Autodesk Inventor part; units mm, degrees
ref_plane "YZ Plane" through (0, 0, 0) normal (1, 0, 0) x (0, 1, 0)
ref_plane "XZ Plane" through (0, 0, 0) normal (0, 1, 0) x (-1, 0, 0)
ref_plane "XY Plane" through (0, 0, 0) normal (0, 0, 1) x (1, 0, 0)
sketch "スケッチ1" plane through (0, 0, 0) normal (0, 0, 1) x (1, 0, 0)
  circle A0 centre (0, 0) radius 30
  circle A1 centre (0, 0) radius 28
  dimension "d0" = 60
  dimension "d21" = 2
extrude "押し出し1" add sketch "スケッチ1" along normal blind 60
sketch "スケッチ6" plane through (0, 0, 0) normal (0, 0, -1) x (-1, 0, 0)
  circle A0 centre (0, 0) radius 28
extrude "押し出し5" add sketch "スケッチ6" against normal blind 2
sketch "スケッチ7" plane through (0, 0, 0) normal (0, 0, -1) x (-1, 0, 0)
  line L0 (0, 0) -> (-30, 0)
  circle A0 centre (0, 0) radius 30
  line L1 (0, 0) -> (0, 30)
  point P0 (-10, -15)
  point P1 (-10, 15)
  point P2 (10, -15)
  point P3 (10, 15)
  dimension "d24" = 20
  dimension "d25" = 30
hole "穴2" at (10, -15, 0) at (10, 15, 0) at (-10, -15, 0) at (-10, 15, 0) direction (0, 0, 1) diameter 3.5 end through all
properties part number "筒"
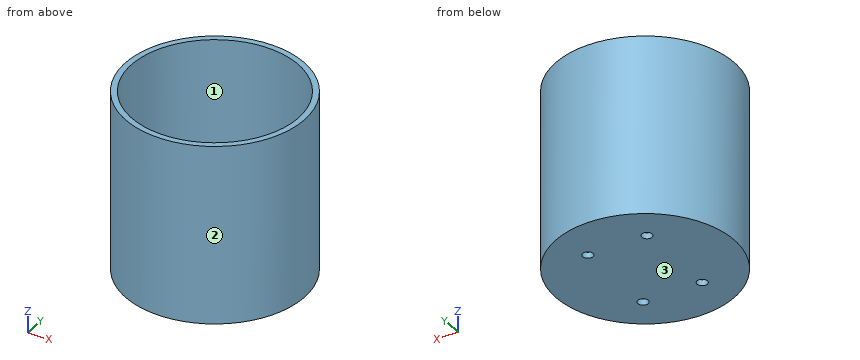
Can you work these out from the model? Positions are in its coordinate system, mm. Face numbers are marked on the shaded views. Coordinates: 2 decimals unless noted, no trailing zeros. Order: outer loops, then holes, each group sorted by start corner. A loop starts at its lowest first (then second) coordinate and runs counter-clockwise, first axis right, second up. Notation, with made-up numbers: (34, -10) - (68, -10) arc R13 ccw to (68, -3) - close; hole circle Ø7 at (15.5, 11.25). An arc over 180 degrees is marked (long way). Answer in a Markdown table with one row per item.
1. If I drill on line 1 along Y through (x, z) = (-10, 1.35); line 2 along X through (y, z) = (15, 0.7); line 3 along Z through (x, y) = (13.5, -17), over which ranges is the centre line in solid material (lowest first)?
Reply:
| item | result |
|---|---|
| line 1 | y = -28.28 to -16.75, -13.25 to 13.25, 16.75 to 28.28 |
| line 2 | x = -25.98 to -11.75, -8.25 to 8.25, 11.75 to 25.98 |
| line 3 | z = 0 to 2 |
2. Suppose I cut it at D-D (z = 53.5). Please give me the cut outline in (x, y), and give its area (3 significant figures).
Reply:
| item | result |
|---|---|
| outline | circle Ø60 at (0, 0); hole circle Ø56 at (0, 0) |
| area | 364 mm^2 |
3. Suppose I cut it at A-A (x = 0). Please give me the cut outline in (y, z), and give its area (3 significant figures).
Reply:
| item | result |
|---|---|
| outline | (-30, 0) - (30, 0) - (30, 60) - (28, 60) - (28, 2) - (-28, 2) - (-28, 60) - (-30, 60) - close |
| area | 352 mm^2 |
4. Suppose I cut it at B-B (x = 10). Please give me the cut outline in (y, z).
Reply:
| item | result |
|---|---|
| outline | (-28.28, 0) - (-16.75, 0) - (-16.75, 2) - (-26.15, 2) - (-26.15, 60) - (-28.28, 60) - close; (-13.25, 0) - (13.25, 0) - (13.25, 2) - (-13.25, 2) - close; (16.75, 0) - (28.28, 0) - (28.28, 60) - (26.15, 60) - (26.15, 2) - (16.75, 2) - close |
5. If we mould it in two halves opening along Y, with no side actions, what happens to the marked faces 1, 2 and 3? For each: pulls with the +Y half, pulls with the -Y half, needs draft (parallel to the pull), parting line crosses it, or undercut.
Reply:
| item | result |
|---|---|
| face 1 | undercut |
| face 2 | parting line crosses it |
| face 3 | needs draft |
6. For pin 1 (12 mm diameter, centred on x = 4, z = 24, fed in from +Y); pin 2 (10 mm diameter, centred on y = 7.5, z = 34, fed in from +X); pin 3 (1 mm diameter, centred on y = 13, z = 9, fed in from -X), each with a flat end and sliding along its axis, tell me the tip position at first contact or that it passes through.
Reply:
| item | result |
|---|---|
| pin 1 | stops at y = 30 |
| pin 2 | stops at x = 29.9 |
| pin 3 | stops at x = -27.27 |
7. Suppose I cut it at C-C (y = 15). Please give me the cut outline in (x, z).
Reply:
| item | result |
|---|---|
| outline | (-25.98, 0) - (-11.75, 0) - (-11.75, 2) - (-23.64, 2) - (-23.64, 60) - (-25.98, 60) - close; (-8.25, 0) - (8.25, 0) - (8.25, 2) - (-8.25, 2) - close; (11.75, 0) - (25.98, 0) - (25.98, 60) - (23.64, 60) - (23.64, 2) - (11.75, 2) - close |
